Part model, mm, in its own coordinate system. A direction names the side the tool comes from. Round coordinates to 2 decimals unless told otherwise and drop trailing zeros. Loops run counter-clockwise (first coordinate to the right, second up) from the corner with the lowest first, then second, coordinate; pieces in that order, holes last. Notation, with made-up numbers: (10.25, 31.25) -> (56.25, 31.25) arc R12 cw to (56.25, 51.25) -> close; hole circle Ø3 at (54, 65.5). An arc over 180 degrees is marked (long way). Answer as a JSON object with one key per item and string values. Group by question number.
from build123d import *

# Parameters (mm, degrees)
BOSS_EXTRUDE2_DEPTH = 4
BOSS_EXTRUDE3_DEPTH = 4
CUT_EXTRUDE1_DEPTH  = 4
SKETCH7_R           = 1
CUT_EXTRUDE2_DEPTH  = 51.104542171
SKETCH9_R           = 1
CUT_EXTRUDE8_DEPTH  = 51.581272683
FILLET1_R           = 10
FILLET2_R           = 10
FILLET3_R           = 3


with BuildPart() as part:
    # Sketch1 → Boss-Extrude2 (new body)
    with BuildSketch(Plane(origin=(0, 0, 0), x_dir=(1, 0, 0), z_dir=(0, 1, 0))):
        with BuildLine():
            Line((5.357809991, 1.999476122), (19.837809991, 13.8))
            Line((19.837809991, 13.8), (42.1, 13.8))
            ThreePointArc((42.1, 13.8), (48.000261939, 7.899738061), (42.1, 1.999476122))
            Line((42.1, 1.999476122), (19.837809991, 1.999476122))
            Line((19.837809991, 1.999476122), (19.837809991, -1.999476122))
            Line((19.837809991, -1.999476122), (5.357809991, -1.999476122))
            Line((5.357809991, -1.999476122), (5.357809991, 1.999476122))
        make_face()
    extrude(amount=BOSS_EXTRUDE2_DEPTH)

    # Sketch4 → Boss-Extrude3 (add)
    with BuildSketch(Plane(origin=(0, 0, 0), x_dir=(-1, 0, 0), z_dir=(0, -1, 0))):
        with BuildLine():
            Line((-19.837809991, 2), (-42.1, 2))
            ThreePointArc((-42.1, 2), (-48, 7.9), (-42.1, 13.8))
            Line((-42.1, 13.8), (-19.837809991, 13.8))
            Line((-19.837809991, 13.8), (-19.837809991, 2))
        make_face()
    extrude(amount=BOSS_EXTRUDE3_DEPTH)

    # Sketch6 → Cut-Extrude1 (cut)
    with BuildSketch(Plane.XZ.offset(4)):
        with BuildLine():
            Line((39.868301502, -4.92331906), (27.984789323, -5.906817464))
            ThreePointArc((27.984789323, -5.906817464), (25.991606786, -7.9), (27.984789323, -9.893182536))
            Line((27.984789323, -9.893182536), (39.867781655, -10.876291126))
            ThreePointArc((39.867781655, -10.876291126), (45.820363894, -7.900324883), (39.868301502, -4.92331906))
        make_face()
    extrude(amount=-CUT_EXTRUDE1_DEPTH, mode=Mode.SUBTRACT)

    # Sketch7 → Cut-Extrude2 (cut, through all)
    with BuildSketch(Plane.XZ):
        with Locations(Location((42.1, -7.9, 0), (0, 0, 270))):
            Circle(SKETCH7_R)
    extrude(amount=-CUT_EXTRUDE2_DEPTH, mode=Mode.SUBTRACT)

    # Sketch9 → Cut-Extrude8 (cut, through all)
    with BuildSketch(Plane(origin=(0, 4, 0), x_dir=(1, 0, 0), z_dir=(0, 1, 0))):
        with Locations(Location((14.5, 0, 0), (0, 0, 270))):
            Circle(SKETCH9_R)
    extrude(amount=-CUT_EXTRUDE8_DEPTH, mode=Mode.SUBTRACT)

    # Fillet1
    # the kernel refuses this fillet: 10 mm, written as the material it takes off along each edge
    with BuildSketch(Plane(origin=(19.837809991, -4, -33.8), x_dir=(1, 0, 0), z_dir=(0, 0, 1))) as fillet1_piece_1:
        with BuildLine():
            CenterArc((8, 10), FILLET1_R, 216.869897646, 53.130102354)
            Line((0, 4), (-0.16, 3.88))
            ThreePointArc((-0.16, 3.88), (-0.2, 2), (-0.2, 0))
            Line((-0.2, 0), (0, -0.2))
            Line((0, -0.2), (8, -0.2))
            Line((8, -0.2), (8, 0))
        make_face()
    extrude(amount=51.8, mode=Mode.SUBTRACT)

    # Fillet2
    fillet2_edges = [part.edges().sort_by_distance(p)[0] for p in [
        (19.837809991, 2, -13.8),
    ]]
    fillet(fillet2_edges, radius=FILLET2_R)

    # Fillet3
    fillet3_edges = [part.edges().sort_by_distance(p)[0] for p in [
        (5.357809991, 4, 0),
        (19.837809991, 4, 0),
    ]]
    fillet(fillet3_edges, radius=FILLET3_R)


solid = part.part
Item 1: Drop flat-ended pins along their axis: pin 1 Ø3 at (x, y) = (25.5, 2.5) entering from +Z; pin 2 Ø0.5 at (y, z) = (0.5, 1) entering from +X. Give the stop position or say it passes through.
Item 2: Band-saw the part on B-B, the plane x = 14.5. List the corners of the cut face in (y, z).
Item 3: Drill centre lines: line 1 (Z direction, x = 42.1, y = -3); line 2 (Z direction, x = 28, y = -3.5); line 3 (X direction, y = 1.2, z = 0). Where is each one in solid material? Low to high.
Item 4: Band-saw the part on A-A, the plane z = 0. List the corners of the cut face in (x, y), plus the area to 3 significant figures.
Item 5: Two-plate mould, pull along Z, no slides. Class faces 1 (the face through (30, 2, -1.999)), 2 (the face through (36, -4, -11)), 3 (the face through (34.01, -2.03, -5.41)): pulls with the +Z half, pulls with the -Z half, needs draft (parallel to the pull), parting line crosses it, or undercut.
Item 6: Band-saw the part on C-C, the plane y = 3.5. List the corners of the cut face in (x, z).
Item 7: Which spindle directions (+Z, -Z, +X, -X, +Y, -Y) get a long thin tool onto all of the face, cutting with end or side? Do faces 4 (the face through (45.82, -2.03, -8.02)), 5 (the face through (13, 2, 1.999)), 6 (the face through (18.98, 3.1, 0.03)). Say none if no direction does.
Entries:
{
 "1": {"pin 1": "z = -2", "pin 2": "x = 19.84"},
 "2": {"outline": "(0, -9.45) -> (4, -9.45) -> (4, -1) -> (0, -1) -> close; (0, 1) -> (4, 1) -> (4, 2) -> (0, 2) -> close"},
 "3": {"line 1": "-13.8 to -11.62, -4.18 to -2", "line 2": "-13.8 to -9.89, -5.91 to -2", "line 3": "5.36 to 13.5, 15.5 to 19.83"},
 "4": {"outline": "(5.36, 0) -> (13.5, 0) -> (13.5, 4) -> (8.36, 4) arc R3 ccw to (5.36, 1) -> close; (15.5, 0) -> (19.84, 0) -> (19.84, 1) arc R3 ccw to (16.84, 4) -> (15.5, 4) -> close", "area": "46.1 mm²"},
 "5": {"face 1": "pulls with the +Z half", "face 2": "needs draft", "face 3": "undercut"},
 "6": {"outline": "(6.7, -3.09) -> (17.08, -11.55) arc R10 ccw to (23.4, -13.8) -> (42.1, -13.8) arc R5.9 ccw to (42.1, -2) -> (18.5, -2) -> (18.5, 2) -> (6.7, 2) -> close; hole circle Ø2 at (14.5, 0); hole circle Ø2 at (42.1, -7.9)"},
 "7": {"face 4": "-Y", "face 5": "+Z, +X, -X, +Y, -Y", "face 6": "+Z, +X, +Y"}
}
